Autodesk Inventor part; units mm, degrees
ref_plane "YZ Plane" through (0, 0, 0) normal (1, 0, 0) x (0, 1, 0)
ref_plane "XZ Plane" through (0, 0, 0) normal (0, 1, 0) x (-1, 0, 0)
ref_plane "XY Plane" through (0, 0, 0) normal (0, 0, 1) x (1, 0, 0)
sketch "Skizze1" plane through (0, 0, 0) normal (1, 0, 0) x (0, 1, 0)
  line L0 (23.95, 0) -> (23.95, 4)
  line L1 (23.95, 4) -> (22.5358, 5.4142)
  line L2 (22.5358, 5.4142) -> (23.95, 6.8284)
  line L3 (23.95, 6.8284) -> (23.95, 26.8284)
  line L4 (23.95, 26.8284) -> (20.25, 26.8284)
  line L5 (20.25, 26.8284) -> (20.25, 30.8284)
  line L6 (20.25, 30.8284) -> (18.25, 30.8284)
  line L7 (18.25, 30.8284) -> (18.25, 0)
  line L8 (18.25, 0) -> (23.95, 0)
  line L9 (0, -6.1657) -> (0, 36.9941)
  point P0 (0, 0)
  dimension "d0" = 4
  dimension "d1" = 2
  dimension "d2" = 135
  dimension "d3" = 20
  dimension "d4" = 23.95
  dimension "d5" = 20.25
  dimension "d6" = 4
  dimension "d7" = 2
revolve "Umdrehung1" add sketch "Skizze1" angle 360 about axis through (0, 0, -10) along (0, 0, 1)
sketch "Skizze2" plane through (0, 0, 26.8284) normal (0, 0, 1) x (1, 0, 0)
  circle A0 centre (0, 0) radius 20.25
  circle A1 centre (0, 0) radius 23.95
extrude "Extrusion1" cut sketch "Skizze2" along normal up to surface (4 mm away) draft 5
properties part number "00_microscope_turret"
Could you check a few things on this model? Use its own coordinates, in mm. A direction names the side the tool comes from. Give positions to 0.01 mm unless a question says otherwise; leave off trailing zeros. Order: outer loops, then holes, each group sorted by start corner. A loop starts at its lowest first (then second) coordinate and runs counter-clockwise, first axis right, second up. Notation, with made-up numbers: (77.5, -23) - (87.5, -23) arc R14 ccw to (87.5, -14) - close; hole circle Ø3 at (83.5, 29.5). An arc over 180 degrees is marked (long way). One line per question, with ' | ' between items. Start each with the question number.
Item 1: I need wall thicknesses on probe 1 along Y at (x, z) = (0, 9); probe 2 along Z at (x, y) = (-4.5, 21). Which ranges of each line are inside material? Lowest first, please. Write a range as [from, to].
Item 2: Thinking about a two-plate mould opening in Z: for faces 3 (the flat face through (6, 18, 30.828)), 4 (the conical face through (15.3, -16.7, 5.3)), 5 (the cylindrical face through (-17.816, -3.956, 15.198)), 6 (the flat face through (18, -5, 0)), which applies, pulls with the +Z half, pulls with the -Z half, needs draft (parallel to the pull), parting line crosses it, or undercut?
Item 3: I'm going to push flat-ended pins straight in: pin 1 Ø10 at (y, z) = (-14.5, 24) entering from +X; pin 2 Ø10 at (x, z) = (7.5, 20) entering from +Y; pin 3 Ø1 at (x, z) = (8.5, 5.5) entering from -Y. Where does each tip first touch, or does it pass through?
Item 4: I want a section at A-A on x = 0. Write out the boundary of the cut face in (y, z), then the cut area to 3 significant figures.
Item 5: I want a section at C-C on z = 8. Write out the boundary of the cut face in (x, y).
Item 6: For faces 1 (the cylindrical face through (23.38, -5.19, 2.03)), 2 (the flat face through (-5, -20, 26.828)), which set-ups out of +Z, -Z, +X, -X, +Y, -Y let a thin tool reach every point of the face, with its end or its side?
Verdict:
1) probe 1: [-23.95, -18.25], [18.25, 23.95] | probe 2: [0, 26.83]
2) face 3: pulls with the +Z half | face 4: undercut | face 5: needs draft | face 6: pulls with the -Z half
3) pin 1: x = 21.99 | pin 2: y = 23.82 | pin 3: y = -21.54
4) outline: (-23.95, 0) - (-18.25, 0) - (-18.25, 30.83) - (-19.9, 30.83) - (-20.25, 26.83) - (-23.95, 26.83) - (-23.95, 6.83) - (-22.54, 5.41) - (-23.95, 4) - close; (18.25, 0) - (23.95, 0) - (23.95, 4) - (22.54, 5.41) - (23.95, 6.83) - (23.95, 26.83) - (20.25, 26.83) - (19.9, 30.83) - (18.25, 30.83) - close | area: 316 mm^2
5) outline: circle Ø47.9 at (0, 0); hole circle Ø36.5 at (0, 0)
6) face 1: +Z, -Z | face 2: +Z
